from build123d import *

# Parameters (mm, degrees)
F0_W     = 7.62
F0_H     = 19.05
F1_DEPTH = 9.525
F2_DEPTH = 50.8
F3_R     = 9.525
F4_DEPTH = 19.051
F5_R     = 9.525
F6_DEPTH = 12.7
F8_DEPTH = 2540
F9_R     = 6.35


with BuildPart() as f1:
    # F0 (on Front) → F1 (new body, symmetric)
    with BuildSketch(Plane.XZ):
        with Locations((3.81, -9.525)):
            Rectangle(F0_W, F0_H)
        with BuildLine():
            Line((7.62, -19.05), (0, -19.05))
            ThreePointArc((0, -19.05), (-25.0864929701, -50.0928763819), (-60.7030030905, -32.0802))
            Line((-60.7030030905, -32.0802), (-68.9011882443, -32.0802))
            ThreePointArc((-68.9011882443, -32.0802), (-25.1411188986, -57.8613332751), (7.62, -19.05))
        make_face()
    extrude(amount=F1_DEPTH, both=True)

    # F0 (on Front) → F2 (join, symmetric)
    with BuildSketch(Plane.XZ):
        Polygon((0, 63.5), (0, 0), (7.62, 0), (19.05, 0), (19.05, 63.5), align=None)
    extrude(amount=F2_DEPTH, both=True)

    # F3 (on Right) → F4 (cut, through all)
    with BuildSketch(Plane.YZ):
        with Locations((25.4, 44.45)):
            Circle(F3_R)
        with Locations((-25.4, 44.45)):
            Circle(F3_R)
    extrude(amount=F4_DEPTH, mode=Mode.SUBTRACT)

    # F5 (on face) → F6 (cut)
    with BuildSketch(Plane(origin=(0, 0, 0), x_dir=(0, -1, 0), z_dir=(-1, 0, 0))):
        with Locations((0, 25.4)):
            Circle(F5_R)
    extrude(amount=-F6_DEPTH, mode=Mode.SUBTRACT)

    # F7 (on Right) → F8 (cut, symmetric)
    with BuildSketch(Plane.YZ):
        with BuildLine():
            ThreePointArc((44.45, 63.5), (48.9401280605, 61.6401280605), (50.8, 57.15))
            Line((50.8, 57.15), (50.8, 63.5))
            Line((50.8, 63.5), (44.45, 63.5))
        make_face()
        with BuildLine():
            Line((-50.8, 63.5), (-50.8, 57.15))
            ThreePointArc((-50.8, 57.15), (-48.9401280605, 61.6401280605), (-44.45, 63.5))
            Line((-44.45, 63.5), (-50.8, 63.5))
        make_face()
        with BuildLine():
            Line((50.8, 0), (50.8, 6.35))
            ThreePointArc((50.8, 6.35), (48.9401280605, 1.8598719395), (44.45, 0))
            Line((44.45, 0), (50.8, 0))
        make_face()
        with BuildLine():
            Line((-50.8, 0), (-44.45, 0))
            ThreePointArc((-44.45, 0), (-48.9401280605, 1.8598719395), (-50.8, 6.35))
            Line((-50.8, 6.35), (-50.8, 0))
        make_face()
    extrude(amount=F8_DEPTH, both=True, mode=Mode.SUBTRACT)

    # F9
    f9_edges = [f1.edges().sort_by_distance(p)[0] for p in [
        (-64.802096, 9.525, -32.0802),
        (-64.802096, -9.525, -32.0802),
    ]]
    fillet(f9_edges, radius=F9_R)


solid = f1.part
The model under review builds one solid part; all positions refer to its coordinate system, in mm. A direction names the side the tool comes from. Round coordinates to 2 decimals unless told otherwise and drop trailing zeros. Order: outer loops, then holes, each group sorted by start corner. A loop starts at its lowest first (then second) coordinate and runs counter-clockwise, first axis right, second up. Notation, with made-up numbers: (41.5, -1) -> (49.5, -1) arc R22 ccw to (49.5, 35) -> close; hole circle Ø6 at (-1.5, 10). An arc over 180 degrees is marked (long way). Write item = value, one per line. Start each with the question number.
Item 1: Consider section D-D on y = 25.4. Write out the cut boundary in (x, z) (3 decimals), plus the area to 3 significant figures.
Item 2: Mouldability with a two-part tool opening along Y and no side actions: class faces 1 (the face through (9.4, -26.6, 53.9)), 2 (the face through (9, 50.8, 32)), 3 (the face through (-18, -9.525, -49)), 4 (the face through (10, -1, 63.5)) as released by +Y, released by -Y, zero draft, split by the parting line, or undercut.
Item 3: Consider section B-B on z = 25.4. Write out the cut boundary in (x, y) (3 decimals).
Item 4: For faces 5 (the face through (-18, 9.525, -49)), 6 (the face through (0, -12, 32)), 7 (the face through (7.62, 0, -10)), 8 (the face through (-64.318, -7.714, -33.99)), 9 (the face through (-64.318, 7.714, -33.99)), list the 3-axis set-ups (+Z, -Z, +X, -X, +Y, -Y) from which the entire face can be reached by the end or side of a thin tool; tool diameter is ignored.
Item 5: Consider section A-A on y = -24. Write out the cut boundary in (x, z).
Item 6: Consider section C-C on y = 0. Write out the cut boundary in (x, z) (3 decimals).
Item 7: For line 1 along Y through (x, z) = (4.5, 44.45) (3 decimals); line 2 along Z through (x, y) = (11, -25); line 3 along X through (y, z) = (-8, -42.5), list the stretches that pass through material, from the lowest coordinate up.
Item 8: Clearance check with flat-ended pins moving along their axes: pin 1 Ø2 at (x, y) = (-42, -11) entering from +Z; pin 2 Ø21 at (x, y) = (13, 3.5) entering from -Z; pin 3 Ø21 at (y, z) = (-0.5, 28) entering from -X; pin 4 Ø7 at (x, y) = (-64, 0.5) entering from +Z. State where each tip first meets the part, or that it passes through.
Conclusion:
q1.outline = (0, 0) -> (19.05, 0) -> (19.05, 34.925) -> (0, 34.925) -> close; (0, 53.975) -> (19.05, 53.975) -> (19.05, 63.5) -> (0, 63.5) -> close
q1.area = 847 mm2
q2.face_1 = undercut
q2.face_2 = released by +Y
q2.face_3 = released by -Y
q2.face_4 = zero draft
q3.outline = (0, -50.8) -> (19.05, -50.8) -> (19.05, 50.8) -> (0, 50.8) -> (0, 9.525) -> (12.7, 9.525) -> (12.7, -9.525) -> (0, -9.525) -> close
q4.face_5 = -Z, +X, -X, +Y
q4.face_6 = +Z, -X, +Y, -Y
q4.face_7 = -Z, +X, +Y, -Y
q4.face_8 = +Z, -X, -Y
q4.face_9 = +Z, -X, +Y
q5.outline = (0, 0) -> (19.05, 0) -> (19.05, 35.03) -> (0, 35.03) -> close; (0, 53.87) -> (19.05, 53.87) -> (19.05, 63.5) -> (0, 63.5) -> close
q6.outline = (-68.901, -32.08) arc R39.37 ccw to (7.62, -19.05) -> (7.62, 0) -> (19.05, 0) -> (19.05, 63.5) -> (0, 63.5) -> (0, 34.925) -> (12.7, 34.925) -> (12.7, 15.875) -> (0, 15.875) -> (0, -19.05) arc R31.75 cw to (-60.703, -32.08) -> close
q7.line_1 = -50.8 to -34.925, -15.875 to 15.875, 34.925 to 50.8
q7.line_2 = 0 to 34.93, 53.97 to 63.5
q7.line_3 = -63.37 to -53.15, -10.35 to -0.13
q8.pin_1 = through
q8.pin_2 = -38.46
q8.pin_3 = 0
q8.pin_4 = -32.08
